The figure shows three views and two pictorial views of one solid part (mm, origin at its lowest corner). Answer the questions. A direction names the side the tool comes from. Coordinates: 2 decimals unless noted, no trailing zeros. Loops run counter-clockwise (first coordinate to the right, second up) from the corner with the lowest first, then second, coordinate; pieces in that order, holes last. Notation, with made-up numbers: M 50.25,-36 L 84.25,-36 A15 cw 84.25,-27 Z; hole C 19.5,71 d7. An arc over 180 degrees is marked long. Answer as a JSON object with one key per item and string values. Group by question number.
1. A cutting plane is placed at B-B on z = 8. Give the vertices of the cut face in (x, y), and give its area (3 significant figures).
2. Straight lines are drawn through the part: L1, parallel to Y at x = 7.5, z = 8; L2, parallel to Z at x = 14.5, y = 10.5; L3, parallel to Z at x = 6.75, y = 12. For each, find the intervals that lie inside material, in ascending order.
3. For the marked faces 1 and 2, determine the directions among +Z, -Z, +X, -X, +Y, -Y from which every point of the face is accessible in a straight line to the end or side of a thin tool.
4. Given pin 1 (2 mm diameter, centred on x = 7, z = 11.5, fed in from -Y); pin 2 (5 mm diameter, centred on x = 8.5, y = 19.5, fed in from +Z); pin 3 (8 mm diameter, centred on y = 63, z = 15.5, fed in from -X), each flat-ended and moving along its own axis, determine where each tip first touches the part or whether it passes through.
5. A cutting plane is placed at A-A on x = 14. Give the vertices of the cut face in (y, z), and give its area (3 significant figures).
6. A cutting plane is placed at D-D on y = 53.5. Give the vertices of the cut face in (x, z).
7. A cutting plane is placed at C-C on y = 88.5. Give the vertices of the cut face in (x, z).
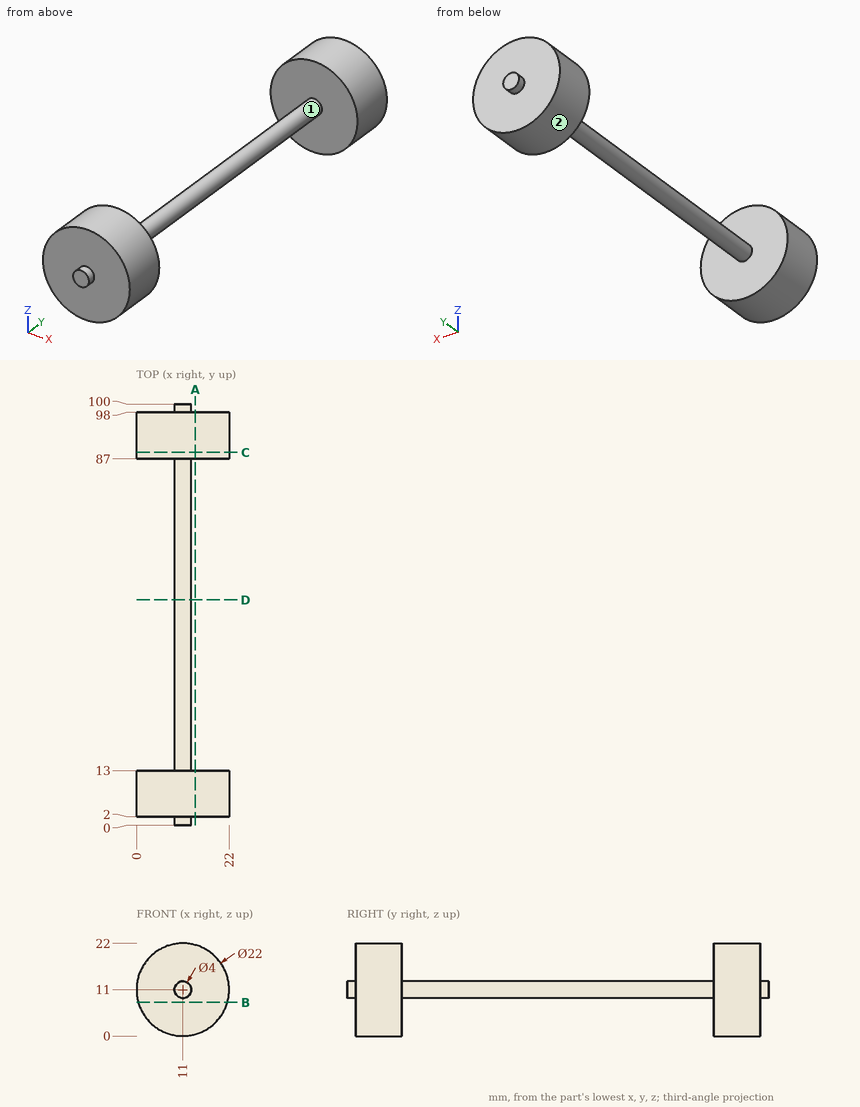
From the geometry:
{
 "1": {"outline": "M 0.42,2 L 21.58,2 L 21.58,13 L 0.42,13 Z; M 0.42,87 L 21.58,87 L 21.58,98 L 0.42,98 Z", "area": "466 mm²"},
 "2": {"L1": "y = 2 to 13, 87 to 98", "L2": "z = 0.57 to 21.43", "L3": "z = 0.85 to 21.15"},
 "3": {"face 1": "none", "face 2": "+Y, -Y"},
 "4": {"pin 1": "stops at y = 2", "pin 2": "stops at z = 13", "pin 3": "stops at x = 9.06"},
 "5": {"outline": "M 2,0.42 L 13,0.42 L 13,21.58 L 2,21.58 Z; M 87,0.42 L 98,0.42 L 98,21.58 L 87,21.58 Z", "area": "466 mm²"},
 "6": {"outline": "C 11,11 d4"},
 "7": {"outline": "C 11,11 d22"}
}
